```python
from build123d import *

# Parameters (mm, degrees)
EXTRUDE_3_DEPTH      = 1374
SKETCH_10_R          = 15.5
CUT_EXTRUDE_11_DEPTH = 1382.439828585


with BuildPart() as part:
    # 草图1 → 拉伸3 (new body)
    with BuildSketch(Plane.XY):
        Polygon((0, 0), (-60, 0), (-60, 120), (0, 120), (0, 130), (-70, 130), (-70, -10), (0, -10), align=None)
    extrude(amount=EXTRUDE_3_DEPTH)

    # 草图10 → 拉伸11 (cut, through all)
    with BuildSketch(Plane(origin=(-60, 0, 0), x_dir=(0, 0, -1), z_dir=(1, 0, 0))):
        with Locations((-45, 60)):
            Circle(SKETCH_10_R)
        with Locations((-135, 60)):
            Circle(SKETCH_10_R)
        with Locations(Location((-1239, 60, 0), (0, 0, 180))):
            Circle(SKETCH_10_R)
        with Locations(Location((-1329, 60, 0), (0, 0, 180))):
            Circle(SKETCH_10_R)
    extrude(amount=-CUT_EXTRUDE_11_DEPTH, mode=Mode.SUBTRACT)


solid = part.part
```
Design review of the part built by this model. Coordinates are the model's own, in mm. A direction names the side the tool comes from. Coordinates: 2 decimals unless noted, no trailing zeros. Order: outer loops, then holes, each group sorted by start corner. A loop starts at its lowest first (then second) coordinate and runs counter-clockwise, first axis right, second up. Notation, with made-up numbers: M 34,49 L 56,49 A19 ccw 56,54 Z; hole C 65.25,26.5 d9. An arc over 180 degrees is marked long. Answer as a JSON object with one key per item and string values. Group by question number.
1) Tool access review of faces 1 (the flat face through (-30, 120, 677)), 2 (the cylindrical face through (-64.93, 59.318, 1223.515)): name each direction out of +Z, -Z, +X, -X, +Y, -Y from which nothing blocks a thin tool from reaching the whole face with its end or side.
2) Wall thickness on L1, parallel to Y at x = -49, z = 519; L2, parallel to Y at x = -65, z = 1239; L3, parallel to X at y = 117.5, z = 954.5: over which ranges is each line inside the solid? List them lowest first.
3) Add section B-B, the plane z = 135. Write out the cut boundary in (x, y), then the cut area to 3 significant figures.
4) Add section A-A, the plane x = -44.5. Write out the cut boundary in (y, z), then the cut area to 3 significant figures.
5) Add section D-D, the plane y = 30. Write out the cut boundary in (x, z).
6) Add section C-C, the plane z = 339. Write out the cut boundary in (x, y).
7) Mouldability with a two-part tool opening along Z and no side actions: class faces 3 (the cylindrical face through (-64.93, 59.318, 1313.515)), 4 (the flat face through (-35, -10, 677)), 5 (the flat face through (-61, 55, 0)) as pulls with the +Z half, pulls with the -Z half, needs draft (parallel to the pull), parting line crosses it, or undercut.
Computed values:
{
 "1": {"face 1": "+Z, -Z, +X", "face 2": "+X, -X"},
 "2": {"L1": "y = -10 to 0, 120 to 130", "L2": "y = -10 to 44.5, 75.5 to 130", "L3": "x = -70 to -60"},
 "3": {"outline": "M -70,-10 L 0,-10 L 0,0 L -60,0 L -60,44.5 L -70,44.5 Z; M -70,75.5 L -60,75.5 L -60,120 L 0,120 L 0,130 L -70,130 Z", "area": "2,290 mm^2"},
 "4": {"outline": "M -10,0 L 0,0 L 0,1374 L -10,1374 Z; M 120,0 L 130,0 L 130,1374 L 120,1374 Z", "area": "27,500 mm^2"},
 "5": {"outline": "M -70,0 L -60,0 L -60,1374 L -70,1374 Z"},
 "6": {"outline": "M -70,-10 L 0,-10 L 0,0 L -60,0 L -60,120 L 0,120 L 0,130 L -70,130 Z"},
 "7": {"face 3": "undercut", "face 4": "needs draft", "face 5": "pulls with the -Z half"}
}
